from build123d import *

# Parameters (mm, degrees)
SKETCH1_W           = 76.2
SKETCH1_H           = 50.8
SKETCH1_R           = 3.1623
SKETCH1_R_2         = 1.4605
BOSS_EXTRUDE1_DEPTH = 1.5875
FILLET1_R           = 2.54


with BuildPart() as part:
    # Sketch1 → Boss-Extrude1 (new body, symmetric)
    with BuildSketch(Plane(origin=(0, 0, 0), x_dir=(1, 0, 0), z_dir=(0, 1, 0))):
        Rectangle(SKETCH1_W, SKETCH1_H)
        with Locations((-25.4, 0)):
            Circle(SKETCH1_R, mode=Mode.SUBTRACT)
        with Locations((25.4, 0)):
            Circle(SKETCH1_R, mode=Mode.SUBTRACT)
        with Locations((0, -20.32)):
            Circle(SKETCH1_R_2, mode=Mode.SUBTRACT)
    extrude(amount=BOSS_EXTRUDE1_DEPTH, both=True)

    # Fillet1
    fillet1_edges = [part.edges().sort_by_distance(p)[0] for p in [
        (-38.1, 0, -25.4),
        (38.1, 0, -25.4),
        (38.1, 0, 25.4),
        (-38.1, 0, 25.4),
    ]]
    fillet(fillet1_edges, radius=FILLET1_R)


solid = part.part
Geometry check sheet. Reference: the model listing, model coordinates, mm. Give positions to 0.01 mm unless a question says otherwise; leave off trailing zeros. Loops run counter-clockwise (first coordinate to the right, second up) from the corner with the lowest first, then second, coordinate; pieces in that order, holes last. Notation, with made-up numbers: M -36.5,9 L -2.5,9 A6 ccw -2.5,17 Z; hole C -10,-10.5 d9. An arc over 180 degrees is marked long. Answer as a JSON object with one key per item and string values. Group by question number.
Item 1: Sectioned sample at C-C on y = 1.05. Record the boundary of the cut face in (x, z).
Item 2: Sectioned sample at D-D on z = 0. Record the boundary of the cut face in (x, y), plus the area to 3 significant figures.
Item 3: Mould release check, pull along X, two halves, no side actions. Record for faces 1 (the cylindrical face through (37.376, -0.022, -24.636)), 2 (the flat face through (-1, 1.588, 0)), 3 (the cylindrical face through (22.24, -0.02, -0.14)): pulls with the +X half, pulls with the -X half, needs draft (parallel to the pull), parting line crosses it, or undercut.
Item 4: Material ranges on L1, parallel to X at y = -0.1, z = 0; L2, parallel to Z at x = 25.4, y = 0.65; L3, parallel to X at y = 1.25, z = -1, recorded low to high.
Item 5: Sectioned sample at A-A on z = 20.32. Record the boundary of the cut face in (x, y).
Item 6: Sectioned sample at B-B on x = -25.4. Record the boundary of the cut face in (y, z).
Findings below:
{
 "1": {"outline": "M -38.1,-22.86 A2.54 ccw -35.56,-25.4 L 35.56,-25.4 A2.54 ccw 38.1,-22.86 L 38.1,22.86 A2.54 ccw 35.56,25.4 L -35.56,25.4 A2.54 ccw -38.1,22.86 Z; hole C -25.4,0 d6.32; hole C 0,20.32 d2.92; hole C 25.4,0 d6.32"},
 "2": {"outline": "M -38.1,-1.59 L -28.56,-1.59 L -28.56,1.59 L -38.1,1.59 Z; M -22.24,-1.59 L 22.24,-1.59 L 22.24,1.59 L -22.24,1.59 Z; M 28.56,-1.59 L 38.1,-1.59 L 38.1,1.59 L 28.56,1.59 Z", "area": "202 mm2"},
 "3": {"face 1": "pulls with the +X half", "face 2": "needs draft", "face 3": "undercut"},
 "4": {"L1": "-38.1 to -28.56, -22.24 to 22.24, 28.56 to 38.1", "L2": "-25.4 to -3.16, 3.16 to 25.4", "L3": "-38.1 to -28.4, -22.4 to 22.4, 28.4 to 38.1"},
 "5": {"outline": "M -38.1,-1.59 L -1.46,-1.59 L -1.46,1.59 L -38.1,1.59 Z; M 1.46,-1.59 L 38.1,-1.59 L 38.1,1.59 L 1.46,1.59 Z"},
 "6": {"outline": "M -1.59,-25.4 L 1.59,-25.4 L 1.59,-3.16 L -1.59,-3.16 Z; M -1.59,3.16 L 1.59,3.16 L 1.59,25.4 L -1.59,25.4 Z"}
}
